from build123d import *

# Parameters (mm, degrees)
F0_R     = 45
F0_R_2   = 15.35
F1_DEPTH = 8
F2_R     = 1
F3_R     = 3
F4_R     = 2


with BuildPart() as f1:
    # F0 (on Top) → F1 (new body)
    with BuildSketch(Plane.XY):
        Circle(F0_R)
        with BuildLine():
            Line((-9.245925, -39.379996), (-9.245925, -37.246354))
            Line((-9.245925, -37.246354), (-4.113387, -40.241164))
            ThreePointArc((-4.113387, -40.241164), (-6.69352, -39.893208), (-9.245925, -39.379996))
        make_face(mode=Mode.SUBTRACT)
        Polygon((-9.245925, -24.436438), (0, -19.098301), (9.245925, -24.436438), (9.245925, -35.112712), (0, -40.45085), (-9.245925, -35.112712), align=None, mode=Mode.SUBTRACT)
        with BuildLine():
            Line((-37.02738, -16.286326), (-32.56624, -20.303154))
            Line((-32.56624, -20.303154), (-34.595454, -20.962485))
            ThreePointArc((-34.595454, -20.962485), (-35.887661, -18.664058), (-37.02738, -16.286326))
        make_face(mode=Mode.SUBTRACT)
        with BuildLine():
            Line((-40.30975, -3.375691), (-38.280536, -2.716359))
            Line((-38.280536, -2.716359), (-39.528641, -8.588233))
            ThreePointArc((-39.528641, -8.588233), (-40.004185, -5.994698), (-40.30975, -3.375691))
        make_face(mode=Mode.SUBTRACT)
        Polygon((-38.471044, -12.5), (-36.251322, -2.057028), (-26.097581, 1.242123), (-18.163563, -5.901699), (-20.383285, -16.344672), (-30.537026, -19.643822), align=None, mode=Mode.SUBTRACT)
        with BuildLine():
            Line((4.047127, -40.247882), (9.245925, -37.246354))
            Line((9.245925, -37.246354), (9.245925, -39.379996))
            ThreePointArc((9.245925, -39.379996), (6.660677, -39.898705), (4.047127, -40.247882))
        make_face(mode=Mode.SUBTRACT)
        with BuildLine():
            Line((34.595454, -20.962485), (32.56624, -20.303154))
            Line((32.56624, -20.303154), (37.279904, -15.699681))
            ThreePointArc((37.279904, -15.699681), (36.033888, -18.380157), (34.595454, -20.962485))
        make_face(mode=Mode.SUBTRACT)
        Polygon((20.383285, -16.344672), (18.163563, -5.901699), (26.097581, 1.242123), (36.251322, -2.057028), (38.471044, -12.5), (30.537026, -19.643822), align=None, mode=Mode.SUBTRACT)
        with BuildLine():
            Line((39.611142, -8.199309), (38.280536, -2.716359))
            Line((38.280536, -2.716359), (40.30975, -3.375691))
            ThreePointArc((40.30975, -3.375691), (40.033162, -5.798031), (39.611142, -8.199309))
        make_face(mode=Mode.SUBTRACT)
        with BuildLine():
            Line((-26.931306, 30.182379), (-29.372968, 24.698315))
            Line((-29.372968, 24.698315), (-30.627092, 26.424468))
            ThreePointArc((-30.627092, 26.424468), (-28.840471, 28.363683), (-26.931306, 30.182379))
        make_face(mode=Mode.SUBTRACT)
        Polygon((-23.776413, 32.725425), (-13.158624, 33.841399), (-6.883267, 25.204112), (-11.225699, 15.45085), (-21.843488, 14.334875), (-28.118845, 22.972163), align=None, mode=Mode.SUBTRACT)
        with BuildLine():
            ThreePointArc((-20.382917, 34.940062), (-18.06327, 36.193778), (-15.666871, 37.293705))
            Line((-15.666871, 37.293705), (-14.412747, 35.567552))
            Line((-14.412747, 35.567552), (-20.382917, 34.940062))
        make_face(mode=Mode.SUBTRACT)
        Circle(F0_R_2, mode=Mode.SUBTRACT)
        Polygon((21.843488, 14.334875), (11.225699, 15.45085), (6.883267, 25.204112), (13.158624, 33.841399), (23.776413, 32.725425), (28.118845, 22.972163), align=None, mode=Mode.SUBTRACT)
        with BuildLine():
            Line((20.339958, 34.965087), (14.412747, 35.567552))
            Line((14.412747, 35.567552), (15.666871, 37.293705))
            ThreePointArc((15.666871, 37.293705), (18.041024, 36.204871), (20.339958, 34.965087))
        make_face(mode=Mode.SUBTRACT)
        with BuildLine():
            Line((30.627092, 26.424468), (29.372968, 24.698315))
            Line((29.372968, 24.698315), (26.931306, 30.182379))
            ThreePointArc((26.931306, 30.182379), (28.840471, 28.363683), (30.627092, 26.424468))
        make_face(mode=Mode.SUBTRACT)
    extrude(amount=F1_DEPTH)

    # F2
    f2_edges = [f1.edges().sort_by_distance(p)[0] for p in [
        (9.054483, 20.327481, 8),
        (10.020946, 29.522756, 8),
        (16.534594, 14.892862, 8),
        (24.981167, 18.653519, 8),
        (25.947629, 27.848794, 8),
        (18.467518, 33.283412, 8),
        (-18.467518, 33.283412, 8),
        (-25.947629, 27.848794, 8),
        (-24.981167, 18.653519, 8),
        (-16.534594, 14.892862, 8),
        (-9.054483, 20.327481, 8),
        (-10.020946, 29.522756, 8),
        (31.174452, -0.407452, 8),
        (22.130572, -2.329788, 8),
        (34.504035, -16.071911, 8),
        (37.361183, -7.278514, 8),
        (19.273424, -11.123186, 8),
        (25.460156, -17.994247, 8),
        (4.622963, -21.767369, 8),
        (-4.622963, -21.767369, 8),
        (-9.245925, -29.774575, 8),
        (9.245925, -29.774575, 8),
        (4.622963, -37.781781, 8),
        (-4.622963, -37.781781, 8),
        (-25.460156, -17.994247, 8),
        (-19.273424, -11.123186, 8),
        (-22.130572, -2.329788, 8),
        (-37.361183, -7.278514, 8),
        (-34.504035, -16.071911, 8),
        (-31.174452, -0.407452, 8),
        (10.020946, 29.522756, 0),
        (18.467518, 33.283412, 0),
        (25.947629, 27.848794, 0),
        (24.981167, 18.653519, 0),
        (16.534594, 14.892862, 0),
        (9.054483, 20.327481, 0),
        (-9.054483, 20.327481, 0),
        (-16.534594, 14.892862, 0),
        (-24.981167, 18.653519, 0),
        (-18.467518, 33.283412, 0),
        (-25.947629, 27.848794, 0),
        (-10.020946, 29.522756, 0),
        (-22.130572, -2.329788, 0),
        (-31.174452, -0.407452, 0),
        (-37.361183, -7.278514, 0),
        (-25.460156, -17.994247, 0),
        (-19.273424, -11.123186, 0),
        (-34.504035, -16.071911, 0),
        (4.622963, -21.767369, 0),
        (-4.622963, -21.767369, 0),
        (-9.245925, -29.774575, 0),
        (-4.622963, -37.781781, 0),
        (4.622963, -37.781781, 0),
        (9.245925, -29.774575, 0),
        (25.460156, -17.994247, 0),
        (34.504035, -16.071911, 0),
        (37.361183, -7.278514, 0),
        (19.273424, -11.123186, 0),
        (22.130572, -2.329788, 0),
        (31.174452, -0.407452, 0),
    ]]
    fillet(f2_edges, radius=F2_R)

    # F3
    f3_edges = [f1.edges().sort_by_distance(p)[0] for p in [
        (-45, 0, 8),
        (-45, 0, 0),
    ]]
    fillet(f3_edges, radius=F3_R)

    # F4
    f4_edges = [f1.edges().sort_by_distance(p)[0] for p in [
        (-15.35, 0, 0),
        (-15.35, 0, 8),
    ]]
    fillet(f4_edges, radius=F4_R)


solid = f1.part
The listing builds one solid part. Answer for the finished solid, in the listing's coordinates (mm). A direction names the side the tool comes from. Coordinates: 2 decimals unless noted, no trailing zeros. Use CSV: the item, a comma, the result in double quotes.
Q1. Given pin 1 Ø1 at (x, y) = (-31, -0.5) entering from -Z; pin 2 Ø18.5 at (x, y) = (0, 0) entering from +Z; pin 3 Ø2.5 at (y, z) = (-38.5, 5) entering from -X; pin 4 Ø2.5 at (y, z) = (-38, 5.5) entering from +X, each flat-ended and moving along its own axis, determine where each tip first touches the part or whether it passes through.
Here are the results:
pin 1,"z = 0.23"
pin 2,"through"
pin 3,"x = -25.25"
pin 4,"x = 25.92"
Q2. Straight lines are drawn through the part: L1, parallel to Y at x = 0, z = 4.2; L2, parallel to Y at x = -34, z = 7; L3, parallel to X at y = -38, z = 5 (3 decimals). For each, find the intervals that lie inside material, in ascending order.
Here are the results:
L1,"-45 to -40.45, -19.1 to -15.35, 15.35 to 45"
L2,"-28.3 to -20.77, -19.01 to -16.53, -1.33 to 28.3"
L3,"-24.104 to -9.246, -7.954 to -4.245, 4.245 to 7.941, 9.246 to 24.104"
Q3. A tool of negligible diameter and unlimited length cuts with its end or side. For faces 1 (the cylindrical face through (-4.837, -37.987, 7.699)), 2 (the cylindrical face through (-16.6, 14.6, 0.3)), 3 (the flat face through (-25.39, -17.97, 3.96)), from which of +Z, -Z, +X, -X, +Y, -Y can it reach the whole face along a straight path? Write none if from no direction.
Here are the results:
face 1,"+Z"
face 2,"-Z"
face 3,"+Z, -Z"
Q4. Section A-A (y = 0) is taken. Give the number of separate pieces and of enclosed holes in the cut face, then the cut area to 3 significant figures.
Here are the results:
separate pieces,"4"
enclosed holes,"0"
area,"376 mm2"
